Autodesk Inventor part; units mm, degrees
ref_plane "YZ Plane" through (0, 0, 0) normal (1, 0, 0) x (0, 1, 0)
ref_plane "XZ Plane" through (0, 0, 0) normal (0, 1, 0) x (-1, 0, 0)
ref_plane "XY Plane" through (0, 0, 0) normal (0, 0, 1) x (1, 0, 0)
sketch "Sketch1" plane through (0, 0, 0) normal (0, 0, 1) x (1, 0, 0)
  line L0 (-4.1988, 5.1716) -> (-7.1858, 8.1586)
  arc A0 (-7.0444, 8.5) -> (-7.1858, 8.1586) centre (-7.0444, 8.3) ccw
  line L1 (-7.0444, 8.5) -> (-4.15, 8.5)
  line L2 (-4.15, 8.5) -> (-4.15, 9)
  arc A1 (-4.15, 9) -> (-5.15, 10) centre (-5.15, 9) ccw
  line L3 (-5.15, 10) -> (-9.6, 10)
  arc A2 (-9.6, 10) -> (-10, 9.6) centre (-9.6, 9.6) ccw
  line L4 (-10, 9.6) -> (-10, 5.15)
  arc A3 (-10, 5.15) -> (-9, 4.15) centre (-9, 5.15) ccw
  line L5 (-9, 4.15) -> (-8.5, 4.15)
  line L6 (-8.5, 4.15) -> (-8.5, 7.0444)
  arc A4 (-8.1586, 7.1858) -> (-8.5, 7.0444) centre (-8.3, 7.0444) ccw
  line L7 (-8.1586, 7.1858) -> (-5.1716, 4.1988)
  arc A5 (-4, 1.3704) -> (-5.1716, 4.1988) centre (-8, 1.3704) ccw
  line L8 (-4, 1.3704) -> (-4, 0)
  line L9 (-4, 0) -> (-4, -1.3704)
  arc A6 (-5.1716, -4.1988) -> (-4, -1.3704) centre (-8, -1.3704) ccw
  line L10 (-5.1716, -4.1988) -> (-8.1586, -7.1858)
  arc A7 (-8.5, -7.0444) -> (-8.1586, -7.1858) centre (-8.3, -7.0444) ccw
  line L11 (-8.5, -7.0444) -> (-8.5, -4.15)
  line L12 (-8.5, -4.15) -> (-9, -4.15)
  arc A8 (-9, -4.15) -> (-10, -5.15) centre (-9, -5.15) ccw
  line L13 (-10, -5.15) -> (-10, -9.6)
  arc A9 (-10, -9.6) -> (-9.6, -10) centre (-9.6, -9.6) ccw
  line L14 (-9.6, -10) -> (-5.15, -10)
  arc A10 (-5.15, -10) -> (-4.15, -9) centre (-5.15, -9) ccw
  line L15 (-4.15, -9) -> (-4.15, -8.5)
  line L16 (-4.15, -8.5) -> (-7.0444, -8.5)
  arc A11 (-7.1858, -8.1586) -> (-7.0444, -8.5) centre (-7.0444, -8.3) ccw
  line L17 (-7.1858, -8.1586) -> (-4.1988, -5.1716)
  arc A12 (-1.3704, -4) -> (-4.1988, -5.1716) centre (-1.3704, -8) ccw
  line L18 (-1.3704, -4) -> (0, -4)
  line L19 (0, -4) -> (1.3704, -4)
  arc A13 (4.1988, -5.1716) -> (1.3704, -4) centre (1.3704, -8) ccw
  line L20 (4.1988, -5.1716) -> (7.1858, -8.1586)
  arc A14 (7.0444, -8.5) -> (7.1858, -8.1586) centre (7.0444, -8.3) ccw
  line L21 (7.0444, -8.5) -> (4.15, -8.5)
  line L22 (4.15, -8.5) -> (4.15, -9)
  arc A15 (4.15, -9) -> (5.15, -10) centre (5.15, -9) ccw
  line L23 (5.15, -10) -> (9.6, -10)
  arc A16 (9.6, -10) -> (10, -9.6) centre (9.6, -9.6) ccw
  line L24 (10, -9.6) -> (10, -5.15)
  arc A17 (10, -5.15) -> (9, -4.15) centre (9, -5.15) ccw
  line L25 (9, -4.15) -> (8.5, -4.15)
  line L26 (8.5, -4.15) -> (8.5, -7.0444)
  arc A18 (8.1586, -7.1858) -> (8.5, -7.0444) centre (8.3, -7.0444) ccw
  line L27 (8.1586, -7.1858) -> (5.1716, -4.1988)
  arc A19 (4, -1.3704) -> (5.1716, -4.1988) centre (8, -1.3704) ccw
  line L28 (4, -1.3704) -> (4, 0)
  line L29 (4, 0) -> (4, 1.3704)
  arc A20 (5.1716, 4.1988) -> (4, 1.3704) centre (8, 1.3704) ccw
  line L30 (5.1716, 4.1988) -> (8.1586, 7.1858)
  arc A21 (8.5, 7.0444) -> (8.1586, 7.1858) centre (8.3, 7.0444) ccw
  line L31 (8.5, 7.0444) -> (8.5, 4.15)
  line L32 (8.5, 4.15) -> (9, 4.15)
  arc A22 (9, 4.15) -> (10, 5.15) centre (9, 5.15) ccw
  line L33 (10, 5.15) -> (10, 9.6)
  arc A23 (10, 9.6) -> (9.6, 10) centre (9.6, 9.6) ccw
  line L34 (9.6, 10) -> (5.15, 10)
  arc A24 (5.15, 10) -> (4.15, 9) centre (5.15, 9) ccw
  line L35 (4.15, 9) -> (4.15, 8.5)
  line L36 (4.15, 8.5) -> (7.0444, 8.5)
  arc A25 (7.1858, 8.1586) -> (7.0444, 8.5) centre (7.0444, 8.3) ccw
  line L37 (7.1858, 8.1586) -> (4.1988, 5.1716)
  arc A26 (1.3704, 4) -> (4.1988, 5.1716) centre (1.3704, 8) ccw
  line L38 (1.3704, 4) -> (0, 4)
  line L39 (0, 4) -> (-1.3704, 4)
  arc A27 (-4.1988, 5.1716) -> (-1.3704, 4) centre (-1.3704, 8) ccw
  circle A28 centre (0, 0) radius 3.05
extrude "Extrusion1" add sketch "Sketch1" along normal mid plane 100
properties part number "Perfil 20 x 20 Básico - LEGP20101" material "Aluminum 6061"
Here's how the part is built. I have some questions about the finished solid (model axes, mm). A direction names the side the tool comes from. Coordinates: 2 decimals unless noted, no trailing zeros. Write each loop counter-clockwise with the first axis right and the second up, starting at its lowest first coordinate (ties: lowest second). Pieces come first, ordered by that corner, then holes. Notation, with made-up numbers: (11.25, 25.25) - (42.25, 25.25) arc R12 cw to (42.25, 48.25) - close; hole circle Ø3 at (-16, 22). An arc over 180 degrees is marked (long way). One line per item, written item: value.
1) We'd pull the mould along Y, two halves only. Please class faces 5 (the flat face through (-2.4, 2.4, 50)), 6 (the flat face through (5.713, 6.686, -0.7)), 7 (the flat face through (6, -8.5, -1)): pulls with the +Y half, pulls with the -Y half, needs draft (parallel to the pull), parting line crosses it, or undercut.
Model answer:
face 5: needs draft
face 6: undercut
face 7: undercut
2) Suppose I cut it at A-A on y = 0. Write out the boundary of the cut face in (x, z), and give its area (3 significant figures).
Model answer:
outline: (-4, -50) - (-3.05, -50) - (-3.05, 50) - (-4, 50) - close; (3.05, -50) - (4, -50) - (4, 50) - (3.05, 50) - close
area: 190 mm²
3) I need wall thicknesses on line 1 along Y through (x, z) = (0, -8.5); line 2 along X through (y, z) = (8.25, 44.5); line 3 along X through (y, z) = (-7, -27). Which ranges of each line are inside material? Lowest first, please.
Model answer:
line 1: y = -4 to -3.05, 3.05 to 4
line 2: x = -10 to -7.24, 7.24 to 10
line 3: x = -10 to -8.5, -7.97 to -6.03, 6.03 to 7.97, 8.5 to 10
4) On a 3-axis mill with a long thin cutter (end or side, diameter ignored), from which of +Z, -Z, +X, -X, +Y, -Y can I reach the whole of each face in a straight line? I mean faces 1 (the flat face through (-4, 0, -1)), 2 (the flat face through (-5.67, 6.64, -0.7)), 3 (the flat face through (4, 0, -1)), 4 (the flat face through (-10, 7, -1)). Say none if no direction works.
Model answer:
face 1: +Z, -Z, -X
face 2: +Z, -Z
face 3: +Z, -Z, +X
face 4: +Z, -Z, -X, +Y, -Y
5) I'm going to push flat-ended pins straight in: P1, Ø1.5, axis at x = 3, z = 24, coming from the -Y side; P2, Ø2, axis at y = 0.5, z = -15, coming from the +X side; P3, Ø3, axis at y = 1.5, z = 15.5, coming from the -X side. Where does each tip first touch, or does it pass through?
Model answer:
P1: stops at y = -4.78
P2: stops at x = 4
P3: stops at x = -4.35
